Here's how the part is built. I have some questions about the finished solid (model axes, mm). Coordinates: 2 decimals unless noted, no trailing zeros. Write each loop counter-clockwise with the first axis right and the second up, starting at its lowest first coordinate (ties: lowest second). Pieces come first, ordered by that corner, then holes.
Item 1: If we section it at A-A (y = 40): Please give me the cut outline in (x, z).
Item 2: I'm going to push flat-ended pins straight in: pin 1 Ø2.5 at (x, y) = (14.61, 13.31) entering from +Z; pin 2 Ø10 at (x, y) = (-15.5, 23.5) entering from -Z. Where does each tip first touch, or does it pass through?
Item 3: If we section it at C-C (z = 1.15): Count the separate pieces of the cut face and the enclosed holes in it, then the cut area to 3 significant figures.
Item 4: If I drill on line 1 (Y direction, x = -37, z = 1.4); line 2 (X direction, y = 41.5, z = 4.5); line 3 (X direction, y = 39.5, z = 1.1), over which ranges is the centre line in solid material (lowest first)?
Item 5: If we section it at B-B (x = 37): Please give me the cut outline in (y, z), then the cut area to 3 significant figures.
from build123d import *

# Parameters (mm, degrees)
SKETCH1_W           = 80
SKETCH1_H           = 50.211199845
SKETCH1_R           = 2.15
BOSS_EXTRUDE1_DEPTH = 5
SKETCH2_R           = 2
CUT_EXTRUDE1_DEPTH  = 10


with BuildPart() as part:
    # Sketch1 → Boss-Extrude1 (new body)
    with BuildSketch(Plane.XY):
        with Locations((0, 25.105599923)):
            Rectangle(SKETCH1_W, SKETCH1_H)
        with Locations((14.610738527, 13.311199845)):
            Circle(SKETCH1_R, mode=Mode.SUBTRACT)
        with Locations((24.810738527, 13.311199845)):
            Circle(SKETCH1_R, mode=Mode.SUBTRACT)
        with Locations((-14.610738527, 13.311199845)):
            Circle(SKETCH1_R, mode=Mode.SUBTRACT)
        with Locations((-24.810738527, 13.311199845)):
            Circle(SKETCH1_R, mode=Mode.SUBTRACT)
    extrude(amount=BOSS_EXTRUDE1_DEPTH)

    # Sketch2 → Cut-Extrude1 (cut)
    with BuildSketch(Plane(origin=(0, 0, 0), x_dir=(-1, 0, 0), z_dir=(0, 0, -1))):
        with Locations((19.710738527, 47.211199845)):
            Circle(SKETCH2_R)
        with Locations((-19.710738527, 47.211199845)):
            Circle(SKETCH2_R)
        with Locations((37, 40)):
            Circle(SKETCH2_R)
        with Locations((-37, 40)):
            Circle(SKETCH2_R)
        with Locations((37, 5)):
            Circle(SKETCH2_R)
        with Locations((-37, 5)):
            Circle(SKETCH2_R)
    extrude(amount=-CUT_EXTRUDE1_DEPTH, mode=Mode.SUBTRACT)


solid = part.part
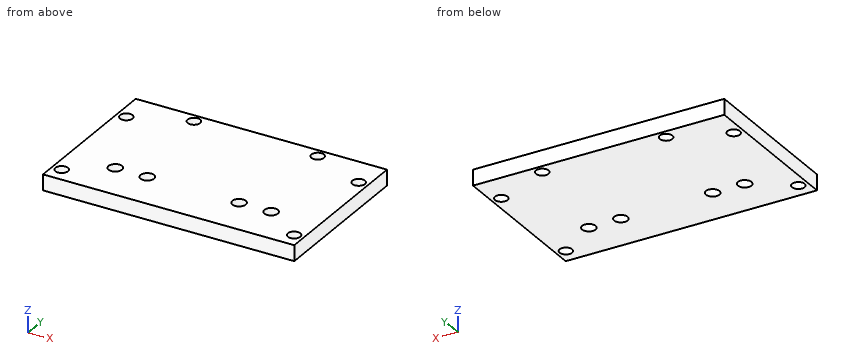
Answer list:
1. outline: (-40, 0) - (-39, 0) - (-39, 5) - (-40, 5) - close; (-35, 0) - (35, 0) - (35, 5) - (-35, 5) - close; (39, 0) - (40, 0) - (40, 5) - (39, 5) - close
2. pin 1: passes through
2. pin 2: stops at z = 0
3. separate pieces: 1
3. enclosed holes: 10
3. area: 3,880 mm2
4. line 1: y = 0 to 3, 7 to 38, 42 to 50.21
4. line 2: x = -40 to -38.32, -35.68 to 35.68, 38.32 to 40
4. line 3: x = -40 to -38.94, -35.06 to 35.06, 38.94 to 40
5. outline: (0, 0) - (3, 0) - (3, 5) - (0, 5) - close; (7, 0) - (38, 0) - (38, 5) - (7, 5) - close; (42, 0) - (50.21, 0) - (50.21, 5) - (42, 5) - close
5. area: 211 mm2
